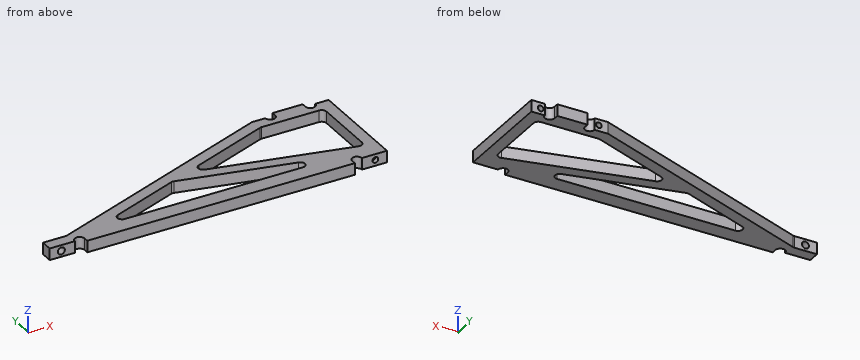
Autodesk Inventor part; units mm, degrees
ref_plane "YZ Plane" through (0, 0, 0) normal (1, 0, 0) x (0, 1, 0)
ref_plane "XZ Plane" through (0, 0, 0) normal (0, 1, 0) x (-1, 0, 0)
ref_plane "XY Plane" through (0, 0, 0) normal (0, 0, 1) x (1, 0, 0)
sketch "スケッチ1" plane through (0, 0, 0) normal (0, 0, 1) x (1, 0, 0)
  line L0 (-72.5, -21.75) -> (72.5, -21.75) construction
  line L1 (72.5, -21.75) -> (72.5, 21.75) construction
  line L2 (72.5, 21.75) -> (-72.5, 21.75) construction
  line L3 (-72.5, 21.75) -> (-72.5, -21.75) construction
  line L4 (-72.5, -21.75) -> (72.5, 21.75) construction
  line L5 (72.5, -21.75) -> (-72.5, 21.75) construction
  line L6 (-67.5, 21.75) -> (-67.5, -21.75) construction
  line L7 (0, 0) -> (0, 21.75) construction
  line L8 (0, 0) -> (-72.5, 0) construction
  line L9 (67.5, 21.75) -> (67.5, -11.6593) construction
  line L10 (-72.5, -21.75) -> (-61.7, -21.75)
  line L11 (49.5, 21.75) -> (49.5, 23.75)
  line L12 (49.5, 23.75) -> (62.5, 23.75)
  line L13 (62.5, 23.75) -> (62.5, 21.75)
  line L14 (66.7, 21.75) -> (72.5, 21.75)
  line L15 (72.5, 21.75) -> (72.5, -21.75)
  line L16 (72.5, -21.75) -> (61.7, -21.75)
  line L17 (-57.5, -21.75) -> (-57.5, -23.75)
  line L18 (-57.5, -23.75) -> (57.5, -23.75)
  line L19 (57.5, -23.75) -> (57.5, -21.75)
  arc A0 (45.3, 21.75) -> (49.5, 21.75) centre (47.4, 21.75) ccw
  arc A1 (62.5, 21.75) -> (66.7, 21.75) centre (64.6, 21.75) ccw
  arc A2 (-57.5, -21.75) -> (-61.7, -21.75) centre (-59.6, -21.75) ccw
  arc A3 (61.7, -21.75) -> (57.5, -21.75) centre (59.6, -21.75) ccw
  line L20 (-72.5, -21.75) -> (-72.5, -16.75)
  line L21 (45.3, 21.75) -> (39.5, 21.75)
  line L22 (66.95, 24.476) -> (70.05, 24.476) construction
  line L23 (70.05, 24.476) -> (70.05, 13.3235) construction
  line L24 (70.05, 13.3235) -> (66.95, 13.3235) construction
  line L25 (66.95, 13.3235) -> (66.95, 24.476) construction
  line L26 (68.5, 24.476) -> (68.5, 13.3235) construction
  line L27 (41.95, 24.476) -> (45.05, 24.476) construction
  line L28 (45.05, 24.476) -> (45.05, 13.9945) construction
  line L29 (45.05, 13.9945) -> (41.95, 13.9945) construction
  line L30 (41.95, 13.9945) -> (41.95, 24.476) construction
  line L31 (43.5, 24.476) -> (43.5, 13.9945) construction
  line L32 (-72.5, -16.75) -> (-62.8649, -16.75)
  line L33 (-62.1586, -16.6211) -> (39.5, 21.75)
  line L34 (40.0708, 16.6211) -> (6.3776, 3.9036) construction
  line L35 (-48.341, -16.75) -> (67.5, -16.75) construction
  line L36 (67.5, -16.75) -> (67.5, 14.75) construction
  line L37 (65.5, 16.75) -> (40.7771, 16.75)
  line L38 (67.5, -16.75) -> (-3.9644, 0) construction
  line L39 (-8.731, -1.7991) -> (-38.085, -12.8789)
  line L40 (-7.5683, -1.7231) -> (39.7036, -12.8028)
  line L41 (39.2472, -16.75) -> (-37.3787, -16.75)
  line L42 (6.6274, 0.0852) -> (65.0436, -13.6065)
  line L43 (67.5, -14.1822) -> (67.5, 16.75)
  arc A4 (65.0436, -13.6065) -> (67.5, -11.6593) centre (65.5, -11.6593) ccw
  arc A5 (6.3776, 3.9036) -> (6.6274, 0.0852) centre (7.0838, 2.0324) ccw
  line L44 (40.0708, 16.6211) -> (6.3776, 3.9036)
  arc A6 (40.7771, 16.75) -> (40.0708, 16.6211) centre (40.7771, 14.75) ccw
  arc A7 (67.5, 14.75) -> (65.5, 16.75) centre (65.5, 14.75) ccw
  arc A8 (-38.085, -12.8789) -> (-37.3787, -16.75) centre (-37.3787, -14.75) ccw
  arc A9 (-7.5683, -1.7231) -> (-8.731, -1.7991) centre (-8.0247, -3.6703) ccw
  arc A10 (39.2472, -16.75) -> (39.7036, -12.8028) centre (39.2472, -14.75) ccw
  arc A11 (-62.8649, -16.75) -> (-62.1586, -16.6211) centre (-62.8649, -14.75) ccw
  point P0 (67.5, -21.75)
  point P1 (-62.5, -16.75)
  point P2 (40.4122, 16.75)
  point P3 (-8.1612, -1.5841)
  point P4 (56.5446, -16.75)
  point P5 (67.5, -11.6593)
  dimension "d16" = 5
  dimension "d20" = 43.5
  dimension "d40" = 135
  dimension "d41" = 10
  dimension "d42" = 2.1
  dimension "d43" = 2
  dimension "d44" = 5
  dimension "d45" = 10
  dimension "d46" = 10
  dimension "d48" = 3.1
  dimension "d50" = 4
  dimension "d51" = 25
  dimension "d52" = 3.1
  dimension "d62" = 6
  dimension "d63" = 6
  dimension "d88" = 10
  dimension "d90" = 5
  dimension "d91" = 5
  dimension "d93" = 5
  dimension "d94" = 94.8651
  dimension "d96" = 47.4325
  dimension "d97" = 2.5
  dimension "d98" = 5
  dimension "d99" = 2
  dimension "d100" = 2
  dimension "d101" = 5
  dimension "d102" = 2
  dimension "d103" = 2
  dimension "d104" = 2
  dimension "d105" = 2
extrude "押し出し1" add sketch "スケッチ1" along normal blind 2.5
mirror "ミラー1" about plane through (0, 0, 0) normal (0, 0, -1) of "押し出し1"
sketch "スケッチ2" plane through (-72.5, -21.75, 2.5) normal (0, -1, 0) x (1, 0, 0)
  line L0 (0, -5) -> (0, 0)
  line L1 (15, -5) -> (130, -5) construction
  line L2 (72.5, -5) -> (72.5, 0) construction
  line L3 (15, 0) -> (130, 0) construction
  point P0 (72.5, -2.5)
  point P1 (140, -2.5)
  point P2 (0, -2.5)
hole "穴1" at (67.5, -21.75, 0) direction (0, 1, 0) diameter 2.459 depth 2
sketch "スケッチ4" plane through (66.7, 21.75, 2.5) normal (0, 1, 0) x (1, 0, 0)
  line L0 (5.8, 5) -> (5.8, 0)
  point P0 (-66.7, 2.5)
  point P1 (1.8, 2.5)
  point P2 (-23.2, 2.5)
  point P3 (5.8, 2.5)
  dimension "d53" = 4
  dimension "d54" = 25
hole "穴2" at (68.5, 21.75, 0) at (43.5, 21.75, 0) direction (0, -1, 0) diameter 2.459 depth 2.5
sketch "スケッチ7" plane through (-72.5, -21.75, 2.5) normal (0, -1, 0) x (1, 0, 0)
  line L0 (0, -5) -> (0, 0)
  line L1 (15, 0) -> (130, 0)
  line L2 (15, -5) -> (130, -5)
  line L3 (0, -2.5) -> (5, -2.5)
  point P0 (72.5, -2.5)
  dimension "d80" = 5
hole "穴3" at (-67.5, -21.75, 0) direction (0, 1, 0) diameter 3 end through all
equation "\"d16\" = d4"
equation "\"d40\" = d6"
equation "\"d41\" = d3"
equation "\"d46\" = d45"
equation "\"d63\" = d62"
properties part number "ForeArm_diagonal" material "アセタール樹脂、黒"
Verification items for the finished model (mm, model axes). Coordinates: 2 decimals unless noted, no trailing zeros. Loops run counter-clockwise (first coordinate to the right, second up) from the corner with the lowest first, then second, coordinate; pieces in that order, holes last. Notation, with made-up numbers: (-34.75, 76) -> (13.25, 76) arc R15 cw to (13.25, 94) -> close; hole circle Ø6 at (-32.75, -37.5). An arc over 180 degrees is marked (long way). Answer as a JSON object with one key per item and string values. Group by question number.
Item 1: Sectioned sample at D-D on x = -41. Record the boundary of the cut face in (y, z).
Item 2: Sectioned sample at A-A on x = -67.5. Record the boundary of the cut face in (y, z), plus the area to 3 significant figures.
Item 3: Sectioned sample at C-C on x = -13.5. Record the boundary of the cut face in (y, z).
Item 4: Sectioned sample at B-B on z = -0.25. State how many separate pieces and enclosed holes the cut face has, plus the area to 3 significant figures.
Item 5: Scan lines: probe 1 along Z at (x, y) = (68.5, 21.15); probe 2 along X at (y, z) = (-20.15, 0); probe 3 along X at (y, z) = (-21.3, 0). Record each from-to range of solid material in increasing order.
Item 6: Depth check by flat-ended pin: pin 1 (1 mm diameter, centred on y = -22.5, z = 1, fed in from -X); pin 2 (6 mm diameter, centred on x = -56.5, y = -9, fed in from +Z); pin 3 (2.5 mm diameter, centred on x = 69, z = -0.5, fed in from +Y); pin 4 (2.5 mm diameter, centred on x = 68, z = 0, fed in from -Y). Enter the tip coordinate at first touch or a pass-through.
Evaluation:
{
 "1": {"outline": "(-23.75, -2.5) -> (-8.63, -2.5) -> (-8.63, 2.5) -> (-23.75, 2.5) -> close"},
 "2": {"outline": "(-21.75, -2.5) -> (-16.75, -2.5) -> (-16.75, -1.5) -> (-21.75, -1.5) -> close; (-21.75, 1.5) -> (-16.75, 1.5) -> (-16.75, 2.5) -> (-21.75, 2.5) -> close", "area": "10.0 mm²"},
 "3": {"outline": "(-23.75, -2.5) -> (-16.75, -2.5) -> (-16.75, 2.5) -> (-23.75, 2.5) -> close; (-3.6, -2.5) -> (1.75, -2.5) -> (1.75, 2.5) -> (-3.6, 2.5) -> close"},
 "4": {"separate pieces": "2", "enclosed holes": "2", "area": "2,170 mm²"},
 "5": {"probe 1": "z = -2.5 to -1.23, 1.23 to 2.5", "probe 2": "x = -72.5 to -69, -66 to -60.96, -58.24 to 58.24, 60.96 to 66.27, 68.73 to 72.5", "probe 3": "x = -72.5 to -69, -66 to -61.65, -57.55 to 57.55, 61.65 to 66.27, 68.73 to 72.5"},
 "6": {"pin 1": "stops at x = -57.5", "pin 2": "passes through", "pin 3": "stops at y = 21.75", "pin 4": "stops at y = -21.75"}
}
